Input: part model. Units: mm. Frame: model coordinates. Face numbers are marked on the shaded views. A direction names the side the tool comes from. Coordinates: 2 decimals unless noted, no trailing zeros. Write each loop counter-clockwise with the first axis right and the second up, starting at its lowest first coordinate (ties: lowest second). Pieces come first, ordered by that corner, then holes. Notation, with made-up numbers: (72.5, 47) - (114.5, 47) arc R33 ccw to (114.5, 82) - close; hole circle Ø2 at (48.25, 75). An arc over 180 degrees is marked (long way). One line per question, with ' | ' between items. Start each with the question number.
1) Section query B-B on y = 71. Return loops of the section in (x, z).
2) Reachability of the marked faces 1 and 2 from +Z, -Z, +X, -X, +Y, -Y: full face, straight path, thin tool, end or side. Return the list, or none.
3) Line query: line 1 (Y direction, x = -12.5, z = -870) (1 decimal); line 2 (X direction, y = 87, z = -878); line 3 (Y direction, x = -20.75, z = -700.5) (3 decimals). Output: solid intervals per line, ascending.
4) First-contact query: P1, Ø0.6, axis at y = 1.5, z = -599.5, coming from the -X side; P2, Ø0.5, axis at y = 10.5, z = -685.5, coming from the +X side; P3, Ø0.6, axis at x = -12.5, z = -317, coming from the -Y side. Flat tips, straight axial feed; report the tip coordinate or a pass-through.
```python
from build123d import *

# Parameters (mm, degrees)
EXTRUDE_THIN1_DEPTH = 1174.75
FILLET1_R           = 1.27


with BuildPart() as part:
    # Sketch1 → Extrude-Thin1 (new body)
    with BuildSketch(Plane.XY):
        with BuildLine():
            Line((0, 0), (-4.7625, 0))
            Line((-4.7625, 0), (-4.7625, 2.38125))
            ThreePointArc((-4.7625, 2.38125), (-9.813894, 4.473606), (-11.90625, 9.525))
            Line((-11.90625, 9.525), (-11.90625, 11.1125))
            Line((-11.90625, 11.1125), (-14.2875, 11.1125))
            Line((-14.2875, 11.1125), (-20.6375, 88.9))
            Line((-20.6375, 88.9), (-22.225, 88.9))
            Line((-22.225, 88.9), (-22.225, 117.475))
            Line((-22.225, 117.475), (0, 117.475))
            Line((0, 117.475), (0, 116.205))
            Line((0, 116.205), (-20.955, 116.205))
            Line((-20.955, 116.205), (-20.955, 90.17))
            Line((-20.955, 90.17), (-19.466949, 90.17))
            Line((-19.466949, 90.17), (-13.116949, 12.3825))
            Line((-13.116949, 12.3825), (-10.63625, 12.3825))
            Line((-10.63625, 12.3825), (-10.63625, 9.525))
            ThreePointArc((-10.63625, 9.525), (-8.439542, 4.944574), (-3.4925, 3.790191))
            Line((-3.4925, 3.790191), (-3.4925, 1.27))
            Line((-3.4925, 1.27), (0, 1.27))
            Line((0, 1.27), (0, 0))
        make_face()
    extrude(amount=-EXTRUDE_THIN1_DEPTH)

    # Fillet1
    fillet1_edges = [part.edges().sort_by_distance(p)[0] for p in [
        (-19.466949, 90.17, -587.375),
        (-10.63625, 12.3825, -587.375),
        (-3.4925, 3.790191, -587.375),
        (-4.7625, 0, -587.375),
        (-14.2875, 11.1125, -587.375),
        (-22.225, 88.9, -587.375),
        (-22.225, 117.475, -587.375),
    ]]
    fillet(fillet1_edges, radius=FILLET1_R)


solid = part.part
```
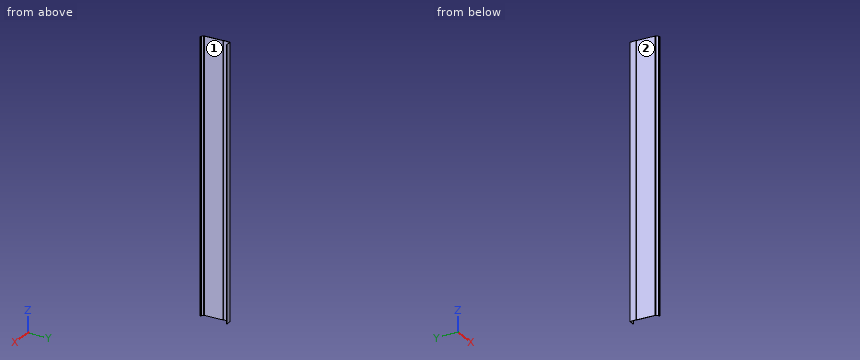
Answer key:
1) outline: (-19.18, -1174.75) - (-17.9, -1174.75) - (-17.9, 0) - (-19.18, 0) - close
2) face 1: +Z, -Z, +X | face 2: +Z, -Z, -X, -Y
3) line 1: 11.1 to 12.4, 116.2 to 117.5 | line 2: -20.48 to -19.21 | line 3: 88.9 to 90.17, 116.205 to 117.475
4) P1: x = -4.76 | P2: x = -10.64 | P3: y = 11.11
